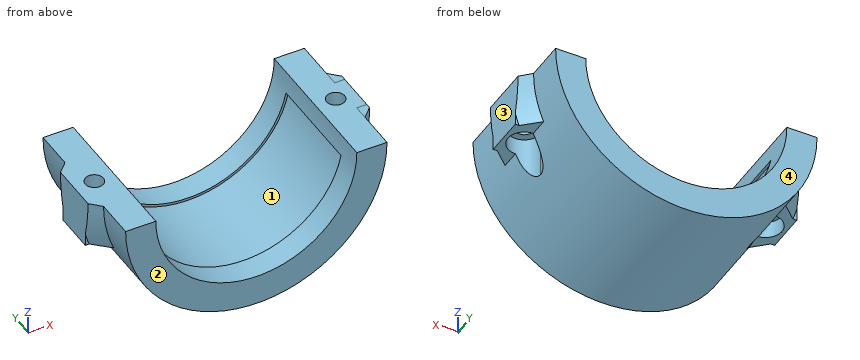
```python
from build123d import *

# Parameters (mm, degrees)
BOSS_EXTRUDE1_DEPTH                          = 30
SKETCH2_W                                    = 8
SKETCH2_H                                    = 8
BOSS_EXTRUDE2_DEPTH                          = 10
CBORE_FOR_M3_HEX_SOCKET_HEAD_CAP_SCR_2_COUNT = 2
CBORE_FOR_M3_HEX_SOCKET_HEAD_CAP_SCR_2_PITCH = 48
SKETCH21_R                                   = 3.25
CUT_EXTRUDE2_DEPTH                           = 46.391188572
CUT_EXTRUDE3_START                           = -25
CUT_EXTRUDE3_DEPTH                           = 20
CHAMFER1_SIZE                                = 3


with BuildPart() as part:
    # Sketch1 → Boss-Extrude1 (new body)
    with BuildSketch(Plane(origin=(0, 0, 0), x_dir=(1, 0, 0), z_dir=(0, 1, 0))):
        with BuildLine():
            Line((26, 0), (20, 0))
            ThreePointArc((20, 0), (0, 20), (-20, 0))
            Line((-20, 0), (-26, 0))
            ThreePointArc((-26, 0), (0, 26), (26, 0))
        make_face()
    extrude(amount=BOSS_EXTRUDE1_DEPTH)

    # Sketch2 → Boss-Extrude2 (add)
    with BuildSketch(Plane.XY):
        with Locations((24, 15)):
            Rectangle(SKETCH2_W, SKETCH2_H)
        with Locations((-24, 15)):
            Rectangle(SKETCH2_W, SKETCH2_H)
    extrude(amount=-BOSS_EXTRUDE2_DEPTH)

    # Sketch20 → CBORE for M3 Hex Socket Head Cap Screw4 (revolve, cut)
    with BuildSketch(Plane(origin=(24, 15, -10), x_dir=(0, 1, 0), z_dir=(1, 0, 0))):
        Polygon((0, 0), (0, 10), (1.8, 10), (1.8, 3.4), (3.25, 3.4), (3.25, 0), align=None)
    cbore_for_m3_hex_socket_head_cap_screw4 = revolve(axis=Axis((24, 15, -16.35), (0, 0, 1)), mode=Mode.SUBTRACT)

    # CBORE for M3 Hex Socket Head Cap Scr 2: CBORE for M3 Hex Socket Head Cap Screw4 ×2
    with Locations(*[(-i * CBORE_FOR_M3_HEX_SOCKET_HEAD_CAP_SCR_2_PITCH, 0, 0) for i in range(1, CBORE_FOR_M3_HEX_SOCKET_HEAD_CAP_SCR_2_COUNT)]):
        add(cbore_for_m3_hex_socket_head_cap_screw4, mode=Mode.SUBTRACT)

    # Sketch21 → Cut-Extrude2 (cut, through all)
    with BuildSketch(Plane(origin=(0, 0, -6.6), x_dir=(-1, 0, 0), z_dir=(0, 0, -1))):
        with Locations((24, 15)):
            Circle(SKETCH21_R)
        with Locations((-24, 15)):
            Circle(SKETCH21_R)
    extrude(amount=CUT_EXTRUDE2_DEPTH, mode=Mode.SUBTRACT)

    # Sketch22 → Cut-Extrude3 (cut)
    with BuildSketch(Plane(origin=(0, 30, 0), x_dir=(1, 0, 0), z_dir=(0, 1, 0)).offset(CUT_EXTRUDE3_START)):
        with BuildLine():
            Line((-20.105969263, 4), (-19.595917942, 4))
            ThreePointArc((-19.595917942, 4), (0, 20), (19.595917942, 4))
            Line((19.595917942, 4), (20.105969263, 4))
            ThreePointArc((20.105969263, 4), (0, 20.5), (-20.105969263, 4))
        make_face()
    extrude(amount=CUT_EXTRUDE3_DEPTH, mode=Mode.SUBTRACT)

    # Chamfer1
    # the kernel refuses this chamfer: 3 mm, written as the material it adds along each edge
    with BuildSketch(Plane(origin=(0, 11, 0), x_dir=(0.7702703819055875, 0, -0.6377174442956852), z_dir=(-0.6377174442956852, 0, -0.7702703819055875))) as chamfer1_piece_1_section:
        Polygon((26, CHAMFER1_SIZE), (26 + CHAMFER1_SIZE, 0), (26, 0), align=None)
    chamfer1_piece_1 = revolve(axis=Axis((0, 11, 0), (0, -1, 0)), revolution_arc=39.621824877, mode=Mode.PRIVATE)
    chamfer1_piece_1 = split(chamfer1_piece_1, bisect_by=Plane(origin=(26.235677781, 9.966963305, -10), z_dir=(0, 0, 1)), keep=Keep.TOP, mode=Mode.PRIVATE)
    chamfer1_piece_1 = split(chamfer1_piece_1, bisect_by=Plane(origin=(28, 9.966963305, -5.200282344), z_dir=(-1, 0, 0)), keep=Keep.TOP, mode=Mode.PRIVATE)
    add(chamfer1_piece_1)
    with BuildSketch(Plane(origin=(0, 19, 0), x_dir=(0.7702703819055875, 0, -0.6377174442956852), z_dir=(-0.6377174442956852, 0, -0.7702703819055875))) as chamfer1_piece_2_section:
        Polygon((26, -CHAMFER1_SIZE), (26 + CHAMFER1_SIZE, 0), (26, 0), align=None)
    chamfer1_piece_2 = revolve(axis=Axis((0, 19, 0), (0, -1, 0)), revolution_arc=39.621824877, mode=Mode.PRIVATE)
    chamfer1_piece_2 = split(chamfer1_piece_2, bisect_by=Plane(origin=(26.235677781, 20.033036695, -10), z_dir=(0, 0, 1)), keep=Keep.TOP, mode=Mode.PRIVATE)
    chamfer1_piece_2 = split(chamfer1_piece_2, bisect_by=Plane(origin=(28, 20.033036695, -5.200282344), z_dir=(-1, 0, 0)), keep=Keep.TOP, mode=Mode.PRIVATE)
    add(chamfer1_piece_2)
    with BuildSketch(Plane(origin=(0, 19, 0), x_dir=(-1, 0, 0), z_dir=(0, 0, 1))) as chamfer1_piece_3_section:
        Polygon((26, -CHAMFER1_SIZE), (26 + CHAMFER1_SIZE, 0), (26, 0), align=None)
    chamfer1_piece_3 = revolve(axis=Axis((0, 19, 0), (0, -1, 0)), revolution_arc=39.621824877, mode=Mode.PRIVATE)
    chamfer1_piece_3 = split(chamfer1_piece_3, bisect_by=Plane(origin=(-26.235677756, 20.033036715, -10), z_dir=(0, 0, 1)), keep=Keep.TOP, mode=Mode.PRIVATE)
    chamfer1_piece_3 = split(chamfer1_piece_3, bisect_by=Plane(origin=(-28, 20.033036715, -5.200282276), z_dir=(1, 0, 0)), keep=Keep.TOP, mode=Mode.PRIVATE)
    add(chamfer1_piece_3)
    with BuildSketch(Plane(origin=(0, 11, 0), x_dir=(-1, 0, 0), z_dir=(0, 0, 1))) as chamfer1_piece_4_section:
        Polygon((26, CHAMFER1_SIZE), (26 + CHAMFER1_SIZE, 0), (26, 0), align=None)
    chamfer1_piece_4 = revolve(axis=Axis((0, 11, 0), (0, -1, 0)), revolution_arc=39.621824877, mode=Mode.PRIVATE)
    chamfer1_piece_4 = split(chamfer1_piece_4, bisect_by=Plane(origin=(-26.235677756, 9.966963285, -10), z_dir=(0, 0, 1)), keep=Keep.TOP, mode=Mode.PRIVATE)
    chamfer1_piece_4 = split(chamfer1_piece_4, bisect_by=Plane(origin=(-28, 9.966963285, -5.200282276), z_dir=(1, 0, 0)), keep=Keep.TOP, mode=Mode.PRIVATE)
    add(chamfer1_piece_4)


solid = part.part
```
Design review of the part built by this model. Coordinates are the model's own, in mm. Face numbers are marked on the shaded views. Give positions to 0.01 mm unless a question says otherwise; leave off trailing zeros. Order: outer loops, then holes, each group sorted by start corner. A loop starts at its lowest first (then second) coordinate and runs counter-clockwise, first axis right, second up. Notation, with made-up numbers: M 32,-31 L 41,-31 A8 cw 41,-23 Z; hole C 12.25,56.25 d3. An arc over 180 degrees is marked long. One line per question, with ' | ' between items. Start each with the question number.
Q1. We need section D-D (z = -4.75). State how many separate pieces and enclosed holes the cut face has, plus the area to 3 significant figures.
Q2. We need section C-C (y = 6). Write out the cut boundary in (x, z), plus the area to 3 significant figures.
Q3. For pin 1 Ø10.5 at (x, y) = (-24, 15) entering from -Z; pin 2 Ø1.5 at (y, z) = (3.5, -9.5) entering from +X; pin 3 Ø0.9 at (x, z) = (28, -9) entering from -Y; pin 4 Ø5 at (x, z) = (-18.5, -5) entering from -Y, all flat-tipped, find the tip position at first contact; note any pin that passes through.
Q4. We need section A-A (x = 0). Write out the cut boundary in (y, z), plus the area to 3 significant figures.
Q5. We need section B-B (z = -12). Write out the cut boundary in (x, y).
Q6. For L1, parallel to Y at x = 24, z = -5; L2, parallel to X at y = 15, z = -9.5; L3, parallel to X at y = 15, z = -2, list the stretches that pass through material, from the lowest coordinate up. Write a range as [from, to].
Q7. The part is to be moulded in two halves that separate along Y. For the marked faces 1, 2, 3 and 4, say which applies: +Y half, -Y half, draft (parallel to the pull), parting line (faces both ways), or undercut.
Returned:
1) separate pieces: 2 | enclosed holes: 2 | area: 384 mm2
2) outline: M -26,0 A26 ccw 26,0 L 20,0 A20 cw 19.6,-4 L 20.11,-4 A20.5 cw -20.11,-4 L -19.6,-4 A20 cw -20,0 Z | area: 406 mm2
3) pin 1: z = -18.01 | pin 2: x = 24.48 | pin 3: y = 10.96 | pin 4: y = 0
4) outline: M 0,-26 L 30,-26 L 30,-20 L 25,-20 L 25,-20.5 L 5,-20.5 L 5,-20 L 0,-20 Z | area: 170 mm2
5) outline: M -23.07,0 L -16,0 L -16,5 L -16.62,5 L -16.62,25 L -16,25 L -16,30 L -23.07,30 L -23.07,18.11 A3.25 cw -23.07,11.89 Z; M 16,0 L 23.07,0 L 23.07,11.89 A3.25 cw 23.07,18.11 L 23.07,30 L 16,30 L 16,25 L 16.62,25 L 16.62,5 L 16,5 Z
6) L1: [0, 13.2], [16.8, 30] | L2: [-28, -27.25], [-20.75, -18.17], [18.17, 20.75], [27.25, 28] | L3: [-28, -25.8], [-22.2, -19.9], [19.9, 22.2], [25.8, 28]
7) face 1: undercut | face 2: -Y half | face 3: draft | face 4: +Y half
